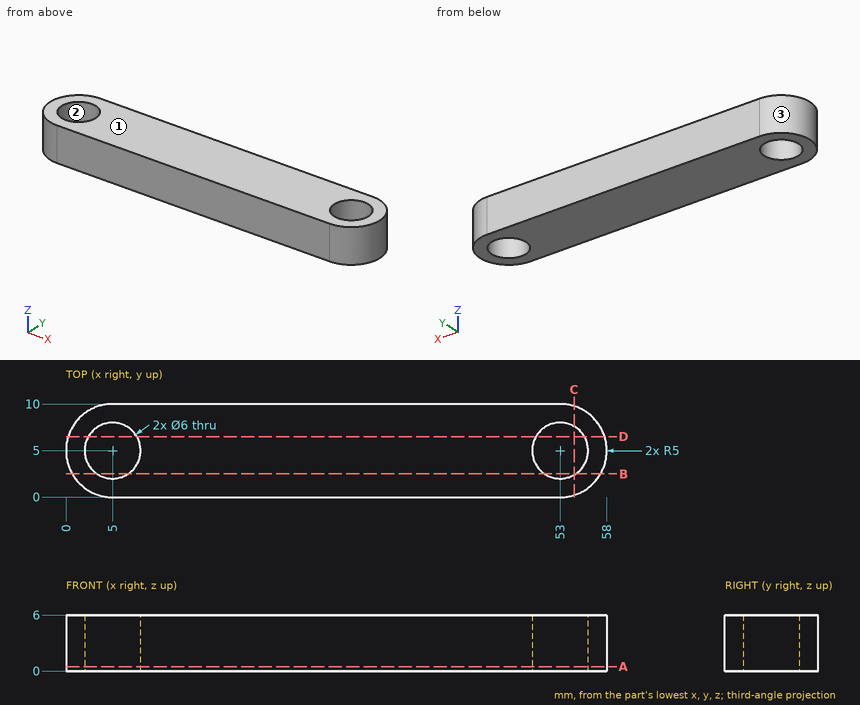
Design review of the part shown in the three views and the two pictorial views. Dimensions are in mm from the part's minimum x, y and z. Give positions to 0.01 mm unless a question says otherwise; leave off trailing zeros. Loops run counter-clockwise (first coordinate to the right, second up) from the corner with the lowest first, then second, coordinate; pieces in that order, holes last. Notation, with made-up numbers: (24, 56) -> (45, 56) arc R18 ccw to (45, 87) -> close; hole circle Ø7 at (10, -40). An arc over 180 degrees is marked (long way). One line per question, with ' | ' between items.
1) The part is to be moulded in two halves that separate along X. For the marked faces 1, 2 and 3, say which applies: +X half, -X half, draft (parallel to the pull), parting line (faces both ways), or undercut.
Resolved:
face 1: draft | face 2: undercut | face 3: -X half
2) We need section D-D (y = 6.5). Write out the cut boundary in (x, z).
Resolved:
outline: (0.23, 0) -> (2.4, 0) -> (2.4, 6) -> (0.23, 6) -> close; (7.6, 0) -> (50.4, 0) -> (50.4, 6) -> (7.6, 6) -> close; (55.6, 0) -> (57.77, 0) -> (57.77, 6) -> (55.6, 6) -> close
3) To check wall thickness, follow probe 1 along X at (y, z) = (3.25, 4.45); probe 2 along X at (y, z) = (4.75, 0.7); probe 3 along Y at (x, z) = (5, 1.5). State the ranges of each line that lie inside material, in increasing order.
Resolved:
probe 1: x = 0.32 to 2.56, 7.44 to 50.56, 55.44 to 57.68 | probe 2: x = 0.01 to 2.01, 7.99 to 50.01, 55.99 to 57.99 | probe 3: y = 0 to 2, 8 to 10
4) Insertion check: pin 1 Ø2 at (y, z) = (8, 1) entering from +X; pin 2 Ø3 at (y, z) = (8.5, 3.5) entering from -X. Each pin has a flat end and moves straight along its axis. Give the tip position at first contact, or say it passes through.
Resolved:
pin 1: stops at x = 57.58 | pin 2: stops at x = 0.42
5) We need section A-A (z = 0.5). Write out the cut boundary in (x, y).
Resolved:
outline: (5, 0) -> (53, 0) arc R5 ccw to (53, 10) -> (5, 10) arc R5 ccw to start; hole circle Ø6 at (5, 5); hole circle Ø6 at (53, 5)
6) We need section B-B (y = 2.5). Write out the cut boundary in (x, z), plus the area to 3 significant figures.
Resolved:
outline: (0.67, 0) -> (3.34, 0) -> (3.34, 6) -> (0.67, 6) -> close; (6.66, 0) -> (51.34, 0) -> (51.34, 6) -> (6.66, 6) -> close; (54.66, 0) -> (57.33, 0) -> (57.33, 6) -> (54.66, 6) -> close | area: 300 mm2
7) We need section C-C (x = 54.5). Write out the cut boundary in (y, z).
Resolved:
outline: (0.23, 0) -> (2.4, 0) -> (2.4, 6) -> (0.23, 6) -> close; (7.6, 0) -> (9.77, 0) -> (9.77, 6) -> (7.6, 6) -> close
